Work out the finished part from the listing and answer in its coordinate system (mm). A direction names the side the tool comes from. Give positions to 0.01 mm unless a question says otherwise; leave off trailing zeros. Loops run counter-clockwise (first coordinate to the right, second up) from the corner with the lowest first, then second, coordinate; pieces in that order, holes last. Notation, with made-up numbers: (70.5, -2.5) - (77.5, -2.5) arc R12 cw to (77.5, 15.5) - close; hole circle Ø1 at (49, 35.5). An arc over 180 degrees is marked (long way). One line per item, written item: value.
from build123d import *


with BuildPart() as part:
    # Sketch1 → Base-Revolve (revolve)
    with BuildSketch(Plane.XY, mode=Mode.PRIVATE) as base_revolve_sk:
        Polygon((0, 0), (0, 22.856406461), (8, 25), (133.7, 25), (140, 23.311920088), (140, 12.5), (137.5, 12.5), (136.345299462, 10.5), (90, 10.5), (83.6909635, 0), align=None)
    revolve(base_revolve_sk.sketch.rotate(Axis((-10, 0, 0), (1, 0, 0)), 90), axis=Axis((-10, 0, 0), (1, 0, 0)))


solid = part.part
1. Section B-B (x = 67.5) is taken. Write down the section's boundary in (y, z), and give its area (3 significant figures).
Output:
outline: circle Ø50 at (0, 0)
area: 1,960 mm²
2. For faces 4 (the flat face through (140, 10, 10)), 5 (the cylindrical face through (138.732, -3.755, 11.923)), determine the directions among +Z, -Z, +X, -X, +Y, -Y from which every point of the face is accessible in a straight line to the end or side of a thin tool.
Output:
face 4: +Z, -Z, +X, +Y, -Y
face 5: +X
3. Section A-A (x = 93) is taken. Write down the section's boundary in (y, z).
Output:
outline: circle Ø50 at (0, 0); hole circle Ø21 at (0, 0)
4. Flat-ended cylindrical pins translate along their axes: pin 1 Ø12 at (x, z) = (16.5, -13) entering from +Y; pin 2 Ø10 at (y, z) = (5.5, 5.5) entering from -X; pin 3 Ø6 at (x, y) = (73.5, 16) entering from +Z; pin 4 Ø1.5 at (x, z) = (115, 14.5) entering from -Y. Find the tip coordinate at first contact, or state that the pin passes through.
Output:
pin 1: stops at y = 24
pin 2: stops at x = 0
pin 3: stops at z = 21.35
pin 4: stops at y = -20.88
5. Find the intervals of material crossed by line 1 along Y through (x, z) = (101, 0); line 2 along Y through (x, z) = (138, 0); line 3 along Z through (x, y) = (69, 1), in increasing order.
Output:
line 1: y = -25 to -10.5, 10.5 to 25
line 2: y = -23.85 to -12.5, 12.5 to 23.85
line 3: z = -24.98 to 24.98
6. The mould has two halves that part along Y. Classify faces 1 (the flat face through (0, 0, 0)), 2 (the cylindrical face through (112.8, -3.2, 10)), 3 (the conical face through (0.5, -6.906, 21.929)): released by +Y, released by -Y, zero draft, split by the parting line, or undercut.
Output:
face 1: zero draft
face 2: undercut
face 3: split by the parting line
